```python
from build123d import *

# Parameters (mm, degrees)
SKETCH1_R                    = 25.4
BOSS_EXTRUDE1_DEPTH          = 76.2
SKETCH2_R                    = 15
CUT_EXTRUDE1_DEPTH           = 25.4
F_12_8_12_8_DIAMETER_HOLE1_D = 32


with BuildPart() as part:
    # Sketch1 → Boss-Extrude1 (new body)
    with BuildSketch(Plane(origin=(0, 0, 0), x_dir=(1, 0, 0), z_dir=(0, 1, 0))):
        with Locations(Location((0, 0, 0), (0, 0, 90))):
            Circle(SKETCH1_R)
    extrude(amount=BOSS_EXTRUDE1_DEPTH)

    # Sketch2 → Cut-Extrude1 (cut)
    with BuildSketch(Plane(origin=(0, 76.2, 0), x_dir=(1, 0, 0), z_dir=(0, 1, 0))):
        with Locations(Location((0, 0, 0), (0, 0, 270))):
            Circle(SKETCH2_R)
    extrude(amount=-CUT_EXTRUDE1_DEPTH, mode=Mode.SUBTRACT)

    # Ø12.8 (12.8) Diameter Hole1 (through all)
    with Locations(Plane(origin=(19.461654008, 25.4, 16.321887859), x_dir=(-0.642594010206, 0, 0.766206850692), z_dir=(0.766206850692, 0, 0.642594010206))):
        with Locations((0, 0)):
            Hole(F_12_8_12_8_DIAMETER_HOLE1_D / 2)


solid = part.part
```
The model under review builds one solid part; all positions refer to its coordinate system, in mm. A direction names the side the tool comes from. Give positions to 0.01 mm unless a question says otherwise; leave off trailing zeros. Write each loop counter-clockwise with the first axis right and the second up, starting at its lowest first coordinate (ties: lowest second). Pieces come first, ordered by that corner, then holes. Notation, with made-up numbers: M -20.75,-10 L 14.25,-10 A10 cw 14.25,-2 Z; hole C 10.5,-36 d10. An arc over 180 degrees is marked long. Answer in a Markdown table with one row per item.
Item 1: For P1, Ø12, axis at x = 14.5, y = 60, coming from the -Z side; P2, Ø1, axis at x = 15, z = 6, coming from the -Y side; P3, Ø8, axis at y = 24.5, z = -17.5, coming from the +X side; P4, Ø12, axis at x = 16.5, y = 24.5, coming from the +Z side, all flat-tipped, find the tip position at first contact; note any pin that passes through.
Check sheet entries:
| item | result |
|---|---|
| P1 | z = -23.94 |
| P2 | y = 0 |
| P3 | x = 21.52 |
| P4 | z = -1.93 |
Item 2: Add section A-A on y = 46.5. Give the boundary of the cut face in (x, z), plus the area to 3 significant figures.
Check sheet entries:
| item | result |
|---|---|
| outline | C 0,0 d50.8 |
| area | 2,030 mm2 |
Item 3: Add section B-B on y = 16.5. Give the boundary of the cut face in (x, z), plus the area to 3 significant figures.
Check sheet entries:
| item | result |
|---|---|
| outline | M -25.13,-3.72 L 8.04,24.09 A25.4 ccw Z; M -8.04,-24.09 A25.4 ccw 25.13,3.72 Z |
| area | 740 mm2 |
Item 4: For line 1 along Y through (x, z) = (-7, -5); line 2 along X through (y, z) = (57, 0); line 3 along Z through (x, y) = (-0.5, 57), list the stretches that pass through material, from the lowest coordinate up.
Check sheet entries:
| item | result |
|---|---|
| line 1 | 0 to 9.41, 41.39 to 50.8 |
| line 2 | -25.4 to -15, 15 to 25.4 |
| line 3 | -25.4 to -14.99, 14.99 to 25.4 |
Item 5: Tool access review of faces 4 (the face through (0, 50.8, 0)), 5 (the face through (11, 76.2, -11)): name each direction out of +Z, -Z, +X, -X, +Y, -Y from which nothing blocks a thin tool from reaching the whole face with its end or side.
Check sheet entries:
| item | result |
|---|---|
| face 4 | +Y |
| face 5 | +Z, -Z, +X, -X, +Y |
Item 6: Add section C-C on y = 36.5. Give the boundary of the cut face in (x, z), plus the area to 3 significant figures.
Check sheet entries:
| item | result |
|---|---|
| outline | M -24.75,-5.72 L 9.94,23.37 A25.4 ccw Z; M -9.94,-23.37 A25.4 ccw 24.75,5.72 Z |
| area | 898 mm2 |
Item 7: Draft analysis for pull direction Z (two halves, no side actions). For faces 1 (the face through (-17.17, 37.57, 18.72)), 2 (the face through (5.255, 11.909, -6.819)), 3 (the face through (0, 0, 0)), state which applies: +Z half, -Z half, draft (parallel to the pull), parting line (faces both ways), or undercut.
Check sheet entries:
| item | result |
|---|---|
| face 1 | parting line |
| face 2 | undercut |
| face 3 | draft |
